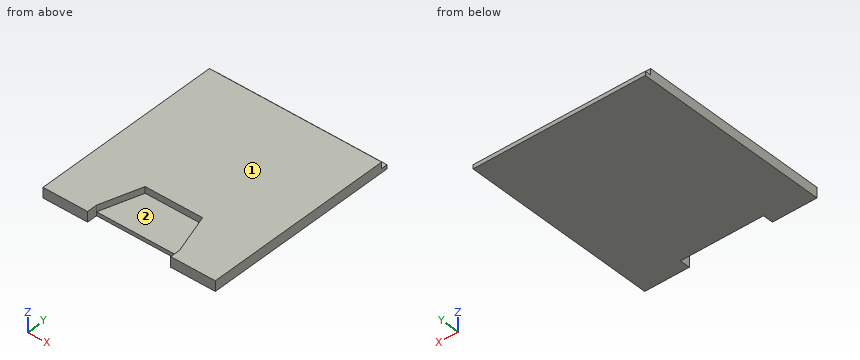
from build123d import *

# Parameters (mm, degrees)
F0_W     = 42.672
F0_H     = 48.768
F1_DEPTH = 2.54
F2_W     = 42.672
F2_H     = 1.54
F3_DEPTH = 1.4986
F4_W     = 20.574
F4_H     = 2.54
F5_DEPTH = 5.08
F7_DEPTH = 1.5875


with BuildPart() as f1:
    # F0 (on Top) → F1 (new body)
    with BuildSketch(Plane.XY):
        Rectangle(F0_W, F0_H)
    extrude(amount=F1_DEPTH)

    # F2 (on face) → F3 (cut)
    with BuildSketch(Plane(origin=(0, 24.384, 0), x_dir=(-1, 0, 0), z_dir=(0, 1, 0))):
        with Locations((0, 1.77)):
            Rectangle(F2_W, F2_H)
    extrude(amount=-F3_DEPTH, mode=Mode.SUBTRACT)

    # F4 (on face) → F5 (cut)
    with BuildSketch(Plane.XY.offset(2.54)):
        with Locations((0, -23.114)):
            Rectangle(F4_W, F4_H)
    extrude(amount=-F5_DEPTH, mode=Mode.SUBTRACT)

    # F6 (on face) → F7 (cut)
    with BuildSketch(Plane.XY.offset(2.54)):
        Polygon((-7.112, -11.684), (-10.287, -21.844), (10.287, -21.844), (7.112, -11.684), align=None)
    extrude(amount=-F7_DEPTH, mode=Mode.SUBTRACT)


solid = f1.part
Part model, mm, in its own coordinate system. Face numbers are marked on the shaded views. Coordinates: 2 decimals unless noted, no trailing zeros. Write each loop counter-clockwise with the first axis right and the second up, starting at its lowest first coordinate (ties: lowest second). Pieces come first, ordered by that corner, then holes. Notation, with made-up numbers: M 59,69.5 L 84,69.5 A20 ccw 84,77.5 Z; hole C 68.25,-20.5 d11. An arc over 180 degrees is marked long. Return JSON: item names as keys, results as strings.
1. Probe L1, parallel to Y at x = 17, z = 1.7; L2, parallel to Z at x = -3, y = -20; L3, parallel to Y at x = 1, z = 2.25. List the from-to ranges inside material, lowest first.
Determined:
{"L1": "-24.38 to 22.89", "L2": "0 to 0.95", "L3": "-11.68 to 22.89"}
2. Saw through at C-C, the plane x = 17.5. Write the cut outline in (y, z), then the cut area to 3 significant figures.
Determined:
{"outline": "M -24.38,0 L 24.38,0 L 24.38,1 L 22.89,1 L 22.89,2.54 L -24.38,2.54 Z", "area": "122 mm²"}
3. Saw through at A-A, the plane z = 0.55. Write the cut outline in (x, y), then the cut area to 3 significant figures.
Determined:
{"outline": "M -21.34,-24.38 L -10.29,-24.38 L -10.29,-21.84 L 10.29,-21.84 L 10.29,-24.38 L 21.34,-24.38 L 21.34,24.38 L -21.34,24.38 Z", "area": "2,030 mm²"}
4. Pull direction X, two halves, no side cores. Call the marked faces 1 and 2: pulls with the +X half, pulls with the -X half, needs draft (parallel to the pull), parting line crosses it, or undercut.
Determined:
{"face 1": "needs draft", "face 2": "undercut"}
5. Saw through at B-B, the plane x = -5.5. Write the cut outline in (y, z), then the cut area to 3 significant figures.
Determined:
{"outline": "M -21.84,0 L 24.38,0 L 24.38,1 L 22.89,1 L 22.89,2.54 L -11.68,2.54 L -11.68,0.95 L -21.84,0.95 Z", "area": "99.0 mm²"}
6. Flat gauge pins, fed straight in: pin 1 Ø8 at (x, y) = (1.5, -17.5) entering from +Z; pin 2 Ø1.2 at (x, z) = (-10.5, 2) entering from +Y. Where does each tip first touch, or does it go through?
Determined:
{"pin 1": "z = 0.95", "pin 2": "y = 22.89"}
